Here's how the part is built. I have some questions about the finished solid (model axes, mm). A direction names the side the tool comes from. Coordinates: 2 decimals unless noted, no trailing zeros. Write each loop counter-clockwise with the first axis right and the second up, starting at its lowest first coordinate (ties: lowest second). Pieces come first, ordered by that corner, then holes. Notation, with made-up numbers: M -27,-23.5 L 1,-23.5 A33 ccw 1,11.5 Z; hole C -35.75,86.25 d2. An arc over 180 degrees is marked long. Write each question's results on one line, items separated by ' | '. Start each with the question number.
Autodesk Fusion 360 part; units mm, degrees
sketch "スケッチ1" plane through (0, 0, 0) normal (0, 0, 1) x (1, 0, 0)
  line L0 (0, 0) -> (74, 0)
  line L1 (74, 0) -> (74, 46)
  line L2 (74, 46) -> (0, 46)
  line L3 (0, 46) -> (0, 0)
  dimension "d1" = 46
  dimension "d2" = 74
extrude "押し出し1" add sketch "スケッチ1" along normal blind 2
sketch "スケッチ2" plane through (0, 0, 2) normal (0, 0, 1) x (-1, 0, 0)
  line L0 (0, -46) -> (0, 0)
  line L1 (0, 0) -> (-74, 0)
  line L2 (-74, 0) -> (-74, -46)
  line L3 (-74, -46) -> (0, -46)
  circle A0 centre (-53, -39) radius 1.6
  circle A1 centre (-53, -39) radius 1.6
  circle A2 centre (-53, -7) radius 1.6
  circle A3 centre (-21, -7) radius 1.6
  circle A4 centre (-21, -39) radius 1.6
  dimension "d5" = 3.2
  dimension "d6" = 7
  dimension "d7" = 21
  dimension "d8" = 3.2
  dimension "d9" = 3.2
  dimension "d10" = 3.2
  dimension "d11" = 3.2
  dimension "d12" = 7
  dimension "d13" = 21
hole "穴1" at (21, 39, 2) at (53, 39, 2) at (53, 7, 2) at (21, 7, 2) direction (0, 0, -1) diameter 3.2 depth 16 tip angle 118
sketch "スケッチ3" plane through (0, 0, 2) normal (0, 0, 1) x (-1, 0, 0)
  circle A0 centre (-53, -7) radius 1.6
  circle A1 centre (-21, -39) radius 1.6
  circle A2 centre (-53, -39) radius 1.6
  circle A3 centre (-21, -7) radius 1.6
  line L0 (0, -46) -> (0, 0)
  line L1 (0, 0) -> (-74, 0)
  line L2 (-74, 0) -> (-74, -46)
  line L3 (-74, -46) -> (0, -46)
  line L4 (-58, -46) -> (-67, -46)
  line L5 (-67, -46) -> (-67, -44)
  line L6 (-67, -44) -> (-58, -44)
  line L7 (-58, -44) -> (-58, -46)
  line L8 (-50, -46) -> (-50, -44)
  line L9 (-41, -46) -> (-50, -46)
  line L10 (-50, -44) -> (-41, -44)
  line L11 (-41, -44) -> (-41, -46)
  line L12 (-33, -46) -> (-33, -44)
  line L13 (-24, -46) -> (-33, -46)
  line L14 (-33, -44) -> (-24, -44)
  line L15 (-24, -44) -> (-24, -46)
  line L16 (-16, -46) -> (-16, -44)
  line L17 (-7, -46) -> (-16, -46)
  line L18 (-16, -44) -> (-7, -44)
  line L19 (-7, -44) -> (-7, -46)
  line L20 (0, -38) -> (-2, -38)
  line L21 (-2, -38) -> (-2, -32)
  line L22 (-2, -32) -> (0, -32)
  line L23 (0, -32) -> (0, -38)
  line L24 (-2, -20) -> (0, -20)
  line L25 (0, -20) -> (0, -26)
  line L26 (-2, -26) -> (-2, -20)
  line L27 (0, -26) -> (-2, -26)
  line L28 (-2, -8) -> (0, -8)
  line L29 (0, -8) -> (0, -14)
  line L30 (-2, -14) -> (-2, -8)
  line L31 (0, -14) -> (-2, -14)
  line L32 (-72, -8) -> (-72, -14)
  line L33 (-72, -38) -> (-74, -38)
  line L34 (-72, -32) -> (-72, -38)
  line L35 (-74, -26) -> (-74, -20)
  line L36 (-74, -32) -> (-72, -32)
  line L37 (-74, -20) -> (-72, -20)
  line L38 (-72, -20) -> (-72, -26)
  line L39 (-74, -14) -> (-74, -8)
  line L40 (-72, -26) -> (-74, -26)
  line L41 (-74, -38) -> (-74, -32)
  line L42 (-74, -8) -> (-72, -8)
  line L43 (-72, -14) -> (-74, -14)
  line L44 (-144, -8) -> (-144, -14)
  line L45 (-144, -38) -> (-146, -38)
  line L46 (-144, -32) -> (-144, -38)
  line L47 (-146, -26) -> (-146, -20)
  line L48 (-146, -32) -> (-144, -32)
  line L49 (-146, -20) -> (-144, -20)
  line L50 (-144, -20) -> (-144, -26)
  line L51 (-146, -14) -> (-146, -8)
  line L52 (-144, -26) -> (-146, -26)
  line L53 (-146, -38) -> (-146, -32)
  line L54 (-146, -8) -> (-144, -8)
  line L55 (-144, -14) -> (-146, -14)
  line L56 (-41, 0) -> (-41, -2)
  line L57 (-67, 0) -> (-58, 0)
  line L58 (-67, -2) -> (-67, 0)
  line L59 (-41, -2) -> (-50, -2)
  line L60 (-7, 0) -> (-7, -2)
  line L61 (-24, 0) -> (-24, -2)
  line L62 (-33, 0) -> (-24, 0)
  line L63 (-50, -2) -> (-50, 0)
  line L64 (-24, -2) -> (-33, -2)
  line L65 (-7, -2) -> (-16, -2)
  line L66 (-58, -2) -> (-67, -2)
  line L67 (-16, -2) -> (-16, 0)
  line L68 (-50, 0) -> (-41, 0)
  line L69 (-58, 0) -> (-58, -2)
  line L70 (-16, 0) -> (-7, 0)
  line L71 (-33, -2) -> (-33, 0)
  line L72 (-41, 44) -> (-41, 42)
  line L73 (-67, 44) -> (-58, 44)
  line L74 (-67, 42) -> (-67, 44)
  line L75 (-41, 42) -> (-50, 42)
  line L76 (-7, 44) -> (-7, 42)
  line L77 (-24, 44) -> (-24, 42)
  line L78 (-33, 44) -> (-24, 44)
  line L79 (-50, 42) -> (-50, 44)
  line L80 (-24, 42) -> (-33, 42)
  line L81 (-7, 42) -> (-16, 42)
  line L82 (-58, 42) -> (-67, 42)
  line L83 (-16, 42) -> (-16, 44)
  line L84 (-50, 44) -> (-41, 44)
  line L85 (-58, 44) -> (-58, 42)
  line L86 (-16, 44) -> (-7, 44)
  line L87 (-33, 42) -> (-33, 44)
  dimension "d17" = 9
  dimension "d18" = 2
  dimension "d19" = 7
  dimension "d22" = 17
  dimension "d23" = 0
  dimension "d24" = 6
  dimension "d25" = 2
  dimension "d26" = 8
  dimension "d29" = 0
  dimension "d30" = 12
  dimension "d33" = -72
  dimension "d34" = 0
  dimension "d37" = 0
  dimension "d38" = 44
extrude "押し出し2" cut sketch "スケッチ3" against normal blind 2 contours L0 L20 L21 L22 L23 | L3 L16 L17 L18 L19 | L0 L24 L25 L26 L27 | L3 L12 L13 L14 L15 | L0 L28 L29 L30 L31 | L3 L8 L9 L10 L11 | L3 L4 L5 L6 L7 | L1 L60 L65 L67 L70 | L1 L61 L62 L64 L71 | L2 L33 L34 L36 L41 | L1 L56 L59 L63 L68 | L2 L35 L37 L38 L40 | L1 L57 L58 L66 L69 | L2 L32 L39 L42 L43
sketch "スケッチ4" plane through (0, 0, 2) normal (0, 0, 1) x (-1, 0, 0)
  line L0 (-50, -2) -> (-50, 0)
  line L1 (-50, 0) -> (-58, 0)
  line L2 (-58, 0) -> (-58, -2)
  line L3 (-58, -2) -> (-67, -2)
  line L4 (-67, -2) -> (-67, 0)
  line L5 (-67, 0) -> (-74, 0)
  line L6 (-74, 0) -> (-74, -8)
  line L7 (-74, -8) -> (-72, -8)
  line L8 (-72, -8) -> (-72, -14)
  line L9 (-72, -14) -> (-74, -14)
  line L10 (-74, -14) -> (-74, -20)
  line L11 (-74, -20) -> (-72, -20)
  line L12 (-72, -20) -> (-72, -26)
  line L13 (-72, -26) -> (-74, -26)
  line L14 (-74, -26) -> (-74, -32)
  line L15 (-74, -32) -> (-72, -32)
  line L16 (-72, -32) -> (-72, -38)
  line L17 (-72, -38) -> (-74, -38)
  line L18 (-74, -38) -> (-74, -46)
  line L19 (-74, -46) -> (-67, -46)
  line L20 (-67, -46) -> (-67, -44)
  line L21 (-67, -44) -> (-58, -44)
  line L22 (-58, -44) -> (-58, -46)
  line L23 (-58, -46) -> (-50, -46)
  line L24 (-50, -46) -> (-50, -44)
  line L25 (-50, -44) -> (-41, -44)
  line L26 (-41, -44) -> (-41, -46)
  line L27 (-41, -46) -> (-33, -46)
  line L28 (-33, -46) -> (-33, -44)
  line L29 (-33, -44) -> (-24, -44)
  line L30 (-24, -44) -> (-24, -46)
  line L31 (-24, -46) -> (-16, -46)
  line L32 (-16, -46) -> (-16, -44)
  line L33 (-16, -44) -> (-7, -44)
  line L34 (-7, -44) -> (-7, -46)
  line L35 (-7, -46) -> (0, -46)
  line L36 (0, -46) -> (0, -38)
  line L37 (0, -38) -> (-2, -38)
  line L38 (-2, -38) -> (-2, -32)
  line L39 (-2, -32) -> (0, -32)
  line L40 (0, -32) -> (0, -26)
  line L41 (0, -26) -> (-2, -26)
  line L42 (-2, -26) -> (-2, -20)
  line L43 (-2, -20) -> (0, -20)
  line L44 (0, -20) -> (0, -14)
  line L45 (0, -14) -> (-2, -14)
  line L46 (-2, -14) -> (-2, -8)
  line L47 (-2, -8) -> (0, -8)
  line L48 (0, -8) -> (0, 0)
  line L49 (0, 0) -> (-7, 0)
  line L50 (-7, 0) -> (-7, -2)
  line L51 (-7, -2) -> (-16, -2)
  line L52 (-16, -2) -> (-16, 0)
  line L53 (-16, 0) -> (-24, 0)
  line L54 (-24, 0) -> (-24, -2)
  line L55 (-24, -2) -> (-33, -2)
  line L56 (-33, -2) -> (-33, 0)
  line L57 (-33, 0) -> (-41, 0)
  line L58 (-41, 0) -> (-41, -2)
  line L59 (-41, -2) -> (-50, -2)
  circle A0 centre (-53, -7) radius 1.6
  circle A1 centre (-21, -39) radius 1.6
  circle A2 centre (-53, -39) radius 1.6
  circle A3 centre (-21, -7) radius 1.6
  circle A4 centre (-37, -23) radius 18
  line L60 (-36, -42) -> (-38, -42)
  line L61 (-38, -42) -> (-38, -4)
  line L62 (-38, -4) -> (-36, -4)
  line L63 (-36, -4) -> (-36, -42)
  line L64 (-41, -42) -> (-43, -42)
  line L65 (-43, -42) -> (-43, -5)
  line L66 (-43, -5) -> (-41, -5)
  line L67 (-41, -5) -> (-41, -42)
  line L68 (-46, -40) -> (-48, -40)
  line L69 (-48, -40) -> (-48, -6)
  line L70 (-48, -6) -> (-46, -6)
  line L71 (-46, -6) -> (-46, -40)
  line L72 (-51, -36) -> (-53, -36)
  line L73 (-53, -36) -> (-53, -11)
  line L74 (-53, -11) -> (-51, -11)
  line L75 (-51, -11) -> (-51, -36)
  line L76 (-33, -42) -> (-31, -42)
  line L77 (-31, -42) -> (-31, -4)
  line L78 (-31, -4) -> (-33, -4)
  line L79 (-33, -4) -> (-33, -42)
  line L80 (-28, -40) -> (-26, -40)
  line L81 (-26, -40) -> (-26, -6)
  line L82 (-26, -6) -> (-28, -6)
  line L83 (-28, -6) -> (-28, -40)
  line L84 (-23, -36) -> (-21, -36)
  line L85 (-21, -36) -> (-21, -11)
  line L86 (-21, -11) -> (-23, -11)
  line L87 (-23, -11) -> (-23, -36)
extrude "押し出し3" cut sketch "スケッチ4" against normal blind 2 contours A4 L85 L87 | A4 L81 L83 | A4 L77 L79 | A4 L61 L63 | A4 L65 L67 | A4 L69 L71 | A4 L73 L75
sketch "スケッチ5" plane through (0, 0, 2) normal (0, 0, 1) x (-1, 0, 0)
  line L0 (-33, -40.5499) -> (-33, -5.4501)
  arc A0 (-31, -6.0294) -> (-33, -5.4501) centre (-37, -23) ccw
  line L1 (-31, -6.0294) -> (-31, -39.9706)
  arc A1 (-33, -40.5499) -> (-31, -39.9706) centre (-37, -23) ccw
  line L2 (-51, -11.6863) -> (-51, -34.3137)
  arc A2 (-53, -31.2462) -> (-51, -34.3137) centre (-37, -23) ccw
  line L3 (-53, -31.2462) -> (-53, -14.7538)
  arc A3 (-51, -11.6863) -> (-53, -14.7538) centre (-37, -23) ccw
  line L4 (-36, -5.0278) -> (-36, -40.9722)
  arc A4 (-38, -40.9722) -> (-36, -40.9722) centre (-37, -23) ccw
  line L5 (-38, -40.9722) -> (-38, -5.0278)
  arc A5 (-36, -5.0278) -> (-38, -5.0278) centre (-37, -23) ccw
  line L6 (-28, -38.5885) -> (-28, -7.4115)
  arc A6 (-26, -8.7522) -> (-28, -7.4115) centre (-37, -23) ccw
  line L7 (-26, -8.7522) -> (-26, -37.2478)
  arc A7 (-28, -38.5885) -> (-26, -37.2478) centre (-37, -23) ccw
  line L8 (-46, -7.4115) -> (-46, -38.5885)
  arc A8 (-48, -37.2478) -> (-46, -38.5885) centre (-37, -23) ccw
  line L9 (-48, -37.2478) -> (-48, -8.7522)
  arc A9 (-46, -7.4115) -> (-48, -8.7522) centre (-37, -23) ccw
  line L10 (-41, -5.4501) -> (-41, -40.5499)
  arc A10 (-43, -39.9706) -> (-41, -40.5499) centre (-37, -23) ccw
  line L11 (-43, -39.9706) -> (-43, -6.0294)
  arc A11 (-41, -5.4501) -> (-43, -6.0294) centre (-37, -23) ccw
  line L12 (-23, -34.3137) -> (-23, -11.6863)
  arc A12 (-21, -14.7538) -> (-23, -11.6863) centre (-37, -23) ccw
  line L13 (-21, -14.7538) -> (-21, -31.2462)
  arc A13 (-23, -34.3137) -> (-21, -31.2462) centre (-37, -23) ccw
  line L14 (-50, -2) -> (-50, 0)
  line L15 (-50, 0) -> (-58, 0)
  line L16 (-58, 0) -> (-58, -2)
  line L17 (-58, -2) -> (-67, -2)
  line L18 (-67, -2) -> (-67, 0)
  line L19 (-67, 0) -> (-74, 0)
  line L20 (-74, 0) -> (-74, -8)
  line L21 (-74, -8) -> (-72, -8)
  line L22 (-72, -8) -> (-72, -14)
  line L23 (-72, -14) -> (-74, -14)
  line L24 (-74, -14) -> (-74, -20)
  line L25 (-74, -20) -> (-72, -20)
  line L26 (-72, -20) -> (-72, -26)
  line L27 (-72, -26) -> (-74, -26)
  line L28 (-74, -26) -> (-74, -32)
  line L29 (-74, -32) -> (-72, -32)
  line L30 (-72, -32) -> (-72, -38)
  line L31 (-72, -38) -> (-74, -38)
  line L32 (-74, -38) -> (-74, -46)
  line L33 (-74, -46) -> (-67, -46)
  line L34 (-67, -46) -> (-67, -44)
  line L35 (-67, -44) -> (-58, -44)
  line L36 (-58, -44) -> (-58, -46)
  line L37 (-58, -46) -> (-50, -46)
  line L38 (-50, -46) -> (-50, -44)
  line L39 (-50, -44) -> (-41, -44)
  line L40 (-41, -44) -> (-41, -46)
  line L41 (-41, -46) -> (-33, -46)
  line L42 (-33, -46) -> (-33, -44)
  line L43 (-33, -44) -> (-24, -44)
  line L44 (-24, -44) -> (-24, -46)
  line L45 (-24, -46) -> (-16, -46)
  line L46 (-16, -46) -> (-16, -44)
  line L47 (-16, -44) -> (-7, -44)
  line L48 (-7, -44) -> (-7, -46)
  line L49 (-7, -46) -> (0, -46)
  line L50 (0, -46) -> (0, -38)
  line L51 (0, -38) -> (-2, -38)
  line L52 (-2, -38) -> (-2, -32)
  line L53 (-2, -32) -> (0, -32)
  line L54 (0, -32) -> (0, -26)
  line L55 (0, -26) -> (-2, -26)
  line L56 (-2, -26) -> (-2, -20)
  line L57 (-2, -20) -> (0, -20)
  line L58 (0, -20) -> (0, -14)
  line L59 (0, -14) -> (-2, -14)
  line L60 (-2, -14) -> (-2, -8)
  line L61 (-2, -8) -> (0, -8)
  line L62 (0, -8) -> (0, 0)
  line L63 (0, 0) -> (-7, 0)
  line L64 (-7, 0) -> (-7, -2)
  line L65 (-7, -2) -> (-16, -2)
  line L66 (-16, -2) -> (-16, 0)
  line L67 (-16, 0) -> (-24, 0)
  line L68 (-24, 0) -> (-24, -2)
  line L69 (-24, -2) -> (-33, -2)
  line L70 (-33, -2) -> (-33, 0)
  line L71 (-33, 0) -> (-41, 0)
  line L72 (-41, 0) -> (-41, -2)
  line L73 (-41, -2) -> (-50, -2)
  circle A14 centre (-53, -7) radius 1.6
  circle A15 centre (-21, -39) radius 1.6
  circle A16 centre (-53, -39) radius 1.6
  circle A17 centre (-21, -7) radius 1.6
1) For faces 4 (the flat face through (73, 38, 1)), 5 (the flat face through (46, 44, 1)), 6 (the flat face through (33, 23, 1)), which set-ups out of +Z, -Z, +X, -X, +Y, -Y let a thin tool reach every point of the face, with its end or its side?
2) For pin 1 Ø0.6 at (y, z) = (16.5, 1) entering from -X; pin 2 Ø1 at (y, z) = (21, 1.5) entering from +X, each with a flat end and sliding along its axis, tell me the tip position at first contact or that it passes through.
3) I want a section at B-B, the plane x = 27. Write out the boundary of the cut face in (y, z), then the cut area to 3 significant figures.
4) I want a section at A-A, the plane y = 17.5. Give the number of separate pieces and of enclosed holes in the cut face, then the cut area to 3 significant figures.
5) We'd pull the mould along Y, two halves only. Please class faces 1 (the flat face through (0, 17, 1)), 2 (the cylindrical face through (19.414, 39.208, 0.986)), 3 (the flat face through (11, 2, 1)): pulls with the +Y half, pulls with the -Y half, needs draft (parallel to the pull), parting line crosses it, or undercut.
6) Please list where these lines run through material, in increasing order: line 1 (X direction, y = 39, z = 0.5); line 2 (Y direction, x = 37, z = 0.55); line 3 (Y direction, x = 27.5, z = 0.85). Write a range as [from, to].
Output:
1) face 4: +Z, -Z, +X | face 5: +Z, -Z, +Y | face 6: +Z, -Z
2) pin 1: stops at x = 0 | pin 2: stops at x = 72
3) outline: M 2,0 L 8.03,0 L 8.03,2 L 2,2 Z; M 37.97,0 L 44,0 L 44,2 L 37.97,2 Z | area: 24.1 mm2
4) separate pieces: 8 | enclosed holes: 0 | area: 120 mm2
5) face 1: needs draft | face 2: undercut | face 3: pulls with the -Y half
6) line 1: x = [0, 19.4], [22.6, 31], [33, 36], [38, 41], [43, 51.4], [54.6, 74] | line 2: y = [0, 5], [41, 46] | line 3: y = [2, 7.71], [38.29, 44]
